Autodesk Inventor part; units mm, degrees
ref_plane "YZ Plane" through (0, 0, 0) normal (1, 0, 0) x (0, 1, 0)
ref_plane "XZ Plane" through (0, 0, 0) normal (0, 1, 0) x (-1, 0, 0)
ref_plane "XY Plane" through (0, 0, 0) normal (0, 0, 1) x (1, 0, 0)
sketch "Sketch1" plane through (0, 0, 0) normal (0, 0, 1) x (1, 0, 0)
  line L0 (0, 0) -> (-10, 0)
  line L1 (-10, 0) -> (-10, 180)
  line L2 (-10, 180) -> (0, 180)
  line L3 (0, 180) -> (0, 0)
  dimension "d0" = 10
  dimension "d1" = 180
extrude "Extrusion1" add sketch "Sketch1" along normal blind 5
sketch "Sketch2" plane through (0, 0, 5) normal (0, 0, 1) x (1, 0, 0)
  line L0 (0, 180) -> (-10, 180)
  line L1 (-10, 0) -> (0, 0)
  line L2 (-10, 180) -> (-10, 0)
  line L3 (0, 0) -> (0, 180)
  point P0 (-5, 172.5)
  point P1 (-5, 7.5)
  dimension "d4" = 7.5
  dimension "d5" = 7.5
  dimension "d8" = 5
  dimension "d9" = 5
hole "Hole1" at (-5, 172.5, 5) at (-5, 7.5, 5) direction (0, 0, -1) diameter 4.5 end through all countersink diameter 9.4 countersink angle 90
properties part number "Pancake_Exit Piece" material "Wood (Birch)"
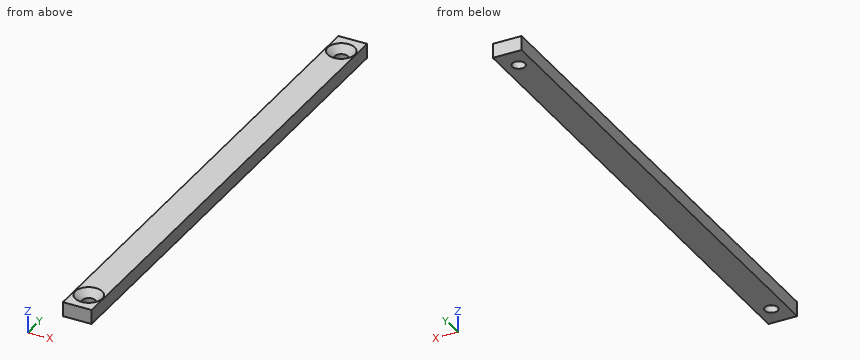
Check sheet for the modelled part. Datum: model origin and axes. Units: mm. Give positions to 0.01 mm unless a question says otherwise; leave off trailing zeros. Loops run counter-clockwise (first coordinate to the right, second up) from the corner with the lowest first, then second, coordinate; pieces in that order, holes last. Notation, with made-up numbers: M 23.25,-26.75 L 74.25,-26.75 A29 ccw 74.25,-5.75 Z; hole C -37.75,68.5 d6. An arc over 180 degrees is marked long. Answer as a JSON object with one key per item and string values. Group by question number.
Q1. Cross-section at A-A on x = -5. Record the cut outline in (y, z), then the cut area to 3 significant figures.
Q2. Cross-section at C-C on z = 1.45. Record the cut outline in (x, y).
Q3. Material ranges on line 1 along Y through (x, z) = (-5, 1.4); line 2 along X through (y, z) = (172.5, 1.45); line 3 along Y through (x, z) = (-6.5, 2.4), recorded low to high. Write a range as [from, to].
Q4. Cross-section at B-B on y = 7.5. Record the cut outline in (x, z).
Evaluation:
{
 "1": {"outline": "M 0,0 L 5.25,0 L 5.25,2.55 L 2.8,5 L 0,5 Z; M 9.75,0 L 170.25,0 L 170.25,2.55 L 167.8,5 L 12.2,5 L 9.75,2.55 Z; M 174.75,0 L 180,0 L 180,5 L 177.2,5 L 174.75,2.55 Z", "area": "843 mm2"},
 "2": {"outline": "M -10,0 L 0,0 L 0,180 L -10,180 Z; hole C -5,7.5 d4.5; hole C -5,172.5 d4.5"},
 "3": {"line 1": "y = [0, 5.25], [9.75, 170.25], [174.75, 180]", "line 2": "x = [-10, -7.25], [-2.75, 0]", "line 3": "y = [0, 5.82], [9.18, 170.82], [174.18, 180]"},
 "4": {"outline": "M -10,0 L -7.25,0 L -7.25,2.55 L -9.7,5 L -10,5 Z; M -2.75,0 L 0,0 L 0,5 L -0.3,5 L -2.75,2.55 Z"}
}
